from build123d import *

# Parameters (mm, degrees)
PAD002_DEPTH  = 33
SKETCH003_W   = 165.06
SKETCH003_H   = 80.96
SKETCH003_W_2 = 23.5
SKETCH003_H_2 = 44.52
PAD003_DEPTH  = 10
SKETCH004_R   = 31
SKETCH004_R_2 = 29.055
PAD004_DEPTH  = 3


with BuildPart() as part:
    # Sketch002 → Pad002 (new body)
    with BuildSketch(Plane.XY):
        with BuildLine():
            ThreePointArc((-22.083648, 12.75), (0, -25.5), (22.083648, 12.75))
            ThreePointArc((-22.083648, 12.75), (0, -28.556543), (22.083648, 12.75))
        make_face()
    extrude(amount=PAD002_DEPTH)

    # Sketch003 → Pad003 (join)
    with BuildSketch(Plane.XY):
        with Locations((0, -11.48)):
            Rectangle(SKETCH003_W, SKETCH003_H)
        with BuildLine():
            ThreePointArc((-6.689544, 7.7), (-10.2, 0), (-6.689544, -7.7))
            Line((-6.689544, -7.7), (6.689544, -7.7))
            ThreePointArc((6.689544, -7.7), (10.2, 0), (6.689544, 7.7))
            Line((-6.689544, 7.7), (6.689544, 7.7))
        make_face(mode=Mode.SUBTRACT)
        with Locations((45, -4.35)):
            Rectangle(SKETCH003_W_2, SKETCH003_H_2, mode=Mode.SUBTRACT)
        with Locations((-45, -4.35)):
            Rectangle(SKETCH003_W_2, SKETCH003_H_2, mode=Mode.SUBTRACT)
    extrude(amount=-PAD003_DEPTH)

    # Sketch004 (on Face3 of Pad003) → Pad004 (join)
    with BuildSketch(Plane.XY):
        with Locations((0, -2)):
            Circle(SKETCH004_R)
        with Locations((0, -2)):
            Circle(SKETCH004_R_2, mode=Mode.SUBTRACT)
    extrude(amount=PAD004_DEPTH)


solid = part.part
Could you check a few things on this model? Use its own coordinates, in mm. A direction names the side the tool comes from. Give positions to 0.01 mm unless a question says otherwise; leave off trailing zeros. Order: outer loops, then holes, each group sorted by start corner. A loop starts at its lowest first (then second) coordinate and runs counter-clockwise, first axis right, second up. Notation, with made-up numbers: (-6, 14) - (1, 14) arc R30 ccw to (1, 45) - close; hole circle Ø7 at (-27, 47). An arc over 180 degrees is marked (long way). One line per question, with ' | ' between items. Start each with the question number.
Item 1: For faces 5 (the flat face through (45, -26.61, -5)), 6 (the flat face through (0, -26, 33)), 7 (the cylindrical face through (-0.75, -25.49, 16.27)), which set-ups out of +Z, -Z, +X, -X, +Y, -Y let a thin tool reach every point of the face, with its end or its side?
Item 2: I need wall thicknesses on probe 1 along Y at (x, z) = (0, 1.95) (3 decimals); probe 2 along Y at (x, z) = (-3.5, 1); probe 3 along Z at (x, y) = (0.5, 26). Which ranges of each line are inside material? Lowest first, please. Write a range as [from, to].
Item 3: I want a section at C-C on y = 22.5. Write out the boundary of the cut face in (x, z).
Item 4: Thinking about a two-plate mould opening in X: for faces 1 (the flat face through (-82.53, -12, -5)), 2 (the flat face through (0, 7.7, -5)), 3 (the flat face through (-1, 29, -5)), 4 (the cylindrical face through (-4.036, 28.736, 1.479)), which applies, pulls with the +X half, pulls with the -X half, needs draft (parallel to the pull), parting line crosses it, or undercut?
Item 5: I want a section at B-B on y = 0. Give the number of separate pieces and of enclosed holes in the cut face, then the cut area to 3 significant figures.
Item 6: I'm going to push flat-ended pins straight in: pin 1 Ø5 at (x, y) = (10, 14.5) entering from +Z; pin 2 Ø3 at (x, z) = (-9.5, 13) entering from -Y; pin 3 Ø8 at (x, y) = (-5.5, 7.5) entering from -Z; pin 4 Ø6 at (y, z) = (-27, 11.5) entering from -X. Where does each tip first touch, or does it pass through?
Item 7: I want a section at D-D on z = 24. Write out the boundary of the cut face in (x, y).
Item 8: I want a section at A-A on z = -6.5. Write out the boundary of the cut face in (x, y).
Verdict:
1) face 5: +Z, -Z | face 6: +Z, +X, -X, +Y, -Y | face 7: +Z
2) probe 1: [-33, -31.055], [-28.557, -25.5], [27.055, 29] | probe 2: [-32.8, -30.84], [-28.32, -25.26], [26.84, 28.8] | probe 3: [-10, 0]
3) outline: (-82.53, -10) - (82.53, -10) - (82.53, 0) - (18.99, 0) - (18.99, 3) - (15.62, 3) - (15.62, 0) - (-15.62, 0) - (-15.62, 3) - (-18.99, 3) - (-18.99, 0) - (-82.53, 0) - close
4) face 1: pulls with the -X half | face 2: undercut | face 3: needs draft | face 4: parting line crosses it
5) separate pieces: 4 | enclosed holes: 0 | area: 1,050 mm^2
6) pin 1: z = 0 | pin 2: y = -27.32 | pin 3: z = -10 | pin 4: x = -14.87
7) outline: (-22.08, 12.75) arc R26.56 ccw (long way) to (22.08, 12.75) arc R25.5 cw (long way) to start
8) outline: (-82.53, -51.96) - (82.53, -51.96) - (82.53, 29) - (-82.53, 29) - close; hole (-56.75, -26.61) - (-33.25, -26.61) - (-33.25, 17.91) - (-56.75, 17.91) - close; hole (-6.69, -7.7) - (6.69, -7.7) arc R10.2 ccw to (6.69, 7.7) - (-6.69, 7.7) arc R10.2 ccw to start; hole (33.25, -26.61) - (56.75, -26.61) - (56.75, 17.91) - (33.25, 17.91) - close
